```python
from build123d import *

# Parameters (mm, degrees)
SKETCH1_W                                           = 336.55
SKETCH1_H                                           = 76.2
SKETCH1_R                                           = 4.7625
SKETCH1_R_2                                         = 3.175
BOSS_EXTRUDE1_DEPTH                                 = 3.175
CSK_FOR_1_4_FLAT_HEAD_MACHINE_SCREW_100_D           = 6.7564
CSK_FOR_1_4_FLAT_HEAD_MACHINE_SCREW_100_CSINK_D     = 12.8778
CSK_FOR_1_4_FLAT_HEAD_MACHINE_SCREW_100_CSINK_ANGLE = 100
SKETCH5_R                                           = 3.175
CUT_EXTRUDE2_DEPTH                                  = 1
CUT_EXTRUDE2_DEPTH_BACK                             = 7.35


with BuildPart() as part:
    # Sketch1 → Boss-Extrude1 (new body, symmetric)
    with BuildSketch(Plane(origin=(0, 0, 0), x_dir=(1, 0, 0), z_dir=(0, 1, 0))):
        with Locations((0, 12.7)):
            Rectangle(SKETCH1_W, SKETCH1_H)
        with Locations((-139.7, -15.875)):
            Circle(SKETCH1_R, mode=Mode.SUBTRACT)
        with Locations((139.7, -15.875)):
            Circle(SKETCH1_R, mode=Mode.SUBTRACT)
        with Locations((131.572, 41.275)):
            Circle(SKETCH1_R_2, mode=Mode.SUBTRACT)
        with Locations((-131.572, 41.275)):
            Circle(SKETCH1_R_2, mode=Mode.SUBTRACT)
    extrude(amount=BOSS_EXTRUDE1_DEPTH, both=True)

    # CSK for 1/4 Flat Head Machine Screw (100)1 (through all)
    with Locations(Plane(origin=(0, 3.175, 0), x_dir=(1, 0, 0), z_dir=(0, 1, 0))):
        with Locations((-131.572, 41.275), (131.572, 41.275)):
            CounterSinkHole(CSK_FOR_1_4_FLAT_HEAD_MACHINE_SCREW_100_D / 2, CSK_FOR_1_4_FLAT_HEAD_MACHINE_SCREW_100_CSINK_D / 2, counter_sink_angle=CSK_FOR_1_4_FLAT_HEAD_MACHINE_SCREW_100_CSINK_ANGLE)

    # Sketch5 → Cut-Extrude2 (cut, two sides)
    with BuildSketch(Plane(origin=(0, 3.175, 0), x_dir=(1, 0, 0), z_dir=(0, 1, 0))) as cut_extrude2_sk:
        with Locations((-114.3, 6.35)):
            Circle(SKETCH5_R)
        with Locations((114.3, 6.35)):
            Circle(SKETCH5_R)
        with Locations((0, 6.35)):
            Circle(SKETCH5_R)
    extrude(amount=CUT_EXTRUDE2_DEPTH, mode=Mode.SUBTRACT)
    extrude(cut_extrude2_sk.sketch, amount=-CUT_EXTRUDE2_DEPTH_BACK, mode=Mode.SUBTRACT)


solid = part.part
```
Input: part model. Units: mm. Frame: model coordinates. Give positions to 0.01 mm unless a question says otherwise; leave off trailing zeros. Write each loop counter-clockwise with the first axis right and the second up, starting at its lowest first coordinate (ties: lowest second). Pieces come first, ordered by that corner, then holes. Notation, with made-up numbers: (-8, 71.5) - (50, 71.5) arc R27 cw to (50, 93.5) - close; hole circle Ø4 at (30, 31.5). An arc over 180 degrees is marked (long way). Write item = value, one per line. Start each with the question number.
1. Section query A-A, the plane z = -6.35. Output: boundary loops of the cut face in (x, y) (3 decimals), then the cut area to 3 significant figures.
2. Mould query, pull axis X, two halves, no side actions, for faces 1 (the flat face through (-168.275, 0, -12)), 2 (the cylindrical face through (128.35, -1.31, -42.29)), 3 (the flat face through (-2, -3.175, -13)). Classes: released by +X, released by -X, zero draft, split by the parting line, or undercut.
3. Section query B-B, the plane x = 114.3. Output: boundary loops of the cut face in (y, z) (3 decimals), then the cut area to 3 significant figures.
4. First-contact query: pin 1 Ø9 at (x, z) = (131.572, -41.275) entering from +Y; pin 2 Ø15 at (x, z) = (139.7, 15.875) entering from -Y (3 decimals). Flat tips, straight axial feed; report the tip coordinate or a pass-through.
5. Ray query, L1, parallel to X at y = 0.5, z = -6.35 (3 decimals); L2, parallel to X at y = -0.25, z = 16 (3 decimals); L3, parallel to X at y = 1, z = -7.5 (3 decimals). Return the intervals inside material, ascending.
Check sheet entries:
q1.outline = (-168.275, -3.175) - (-117.475, -3.175) - (-117.475, 3.175) - (-168.275, 3.175) - close; (-111.125, -3.175) - (-3.175, -3.175) - (-3.175, 3.175) - (-111.125, 3.175) - close; (3.175, -3.175) - (111.125, -3.175) - (111.125, 3.175) - (3.175, 3.175) - close; (117.475, -3.175) - (168.275, -3.175) - (168.275, 3.175) - (117.475, 3.175) - close
q1.area = 2,020 mm2
q2.face_1 = released by -X
q2.face_2 = undercut
q2.face_3 = zero draft
q3.outline = (-3.175, -50.8) - (3.175, -50.8) - (3.175, -9.525) - (-3.175, -9.525) - close; (-3.175, -3.175) - (3.175, -3.175) - (3.175, 25.4) - (-3.175, 25.4) - close
q3.area = 444 mm2
q4.pin_1 = 1.55
q4.pin_2 = -3.175
q5.L1 = -168.275 to -117.475, -111.125 to -3.175, 3.175 to 111.125, 117.475 to 168.275
q5.L2 = -168.275 to -144.461, -134.939 to 134.939, 144.461 to 168.275
q5.L3 = -168.275 to -117.259, -111.341 to -2.959, 2.959 to 111.341, 117.259 to 168.275
